Part model, mm, in its own coordinate system. A direction names the side the tool comes from. Coordinates: 2 decimals unless noted, no trailing zeros. Order: outer loops, then holes, each group sorted by start corner. A loop starts at its lowest first (then second) coordinate and runs counter-clockwise, first axis right, second up. Notation, with made-up numbers: (-33, 63) - (19, 63) arc R13 cw to (19, 82) - close; hole circle Ø4 at (84.25, -13.5). An arc over 180 degrees is marked (long way). Use a Markdown table: item, result. Add a question column.
1) Drop flat-ended pins along their axis: P1, Ø1, axis at y = 1.5, z = -1.5, coming from the -X side; P2, Ø3, axis at x = -2.5, y = -2, coming from the -Z side; P3, Ø5, axis at y = 3.5, z = -2, coming from the +X side. Give the stop position or say it passes through.
2) Wall check: L1, parallel to Z at x = 4.5, y = -4.5; L2, parallel to Z at x = -4, y = 2.5; L3, parallel to Z at x = -6.75, y = 1.25. Give the ranges that are in metal, low to high. Write a range as [from, to].
3) Two-plate mould, pull along Z, no slides. Class faces 5 (the face through (0, -5.5, -3)), 6 (the face through (4.52, -1.15, -6)), 7 (the face through (7.324, 0.077, -4.541)): +Z half, -Z half, draft (parallel to the pull), parting line (faces both ways), or undercut.
4) Tool access for faces 1 (the face through (-1.08, 4.88, -12.48)), 2 (the face through (-9.866, -2.835, -1.154)), 3 (the face through (9.884, -2.835, -1.154)), 4 (the face through (3.233, 1.341, -9.986)): list every direction of +Z, -Z, +X, -X, +Y, -Y with a clear straight run to the whole face (end or side of a thin tool).
5) Saw through at B-B on z = -4.75. List the corners of the cut face in (x, y), then the cut area to 3 significant figures.
6) Saw through at A-A on z = -1.5. List the corners of the cut face in (x, y).
```python
from build123d import *

# Parameters (mm, degrees)
Y_KSEKLIK_EKSTR_ZYON1_DEPTH = 5.5
IZIM4_R                     = 0.75
Y_KSEKLIK_EKSTR_ZYON2_DEPTH = 10.5
RADYUS1_R                   = 0.1
RADYUS2_R                   = 1.4


with BuildPart() as part:
    # Çizim1 → Yükseklik-Ekstrüzyon1 (new, symmetric)
    with BuildSketch(Plane(origin=(0, 0, 0), x_dir=(1, 0, 0), z_dir=(0, 1, 0))):
        Polygon((-9.25, 0), (9.25, 0), (9.25, 3), (5.5, 6), (-5.5, 6), (-9.25, 3), align=None)
    extrude(amount=Y_KSEKLIK_EKSTR_ZYON1_DEPTH, both=True)

    # Çizim2 → Döndür1 (revolve)
    with BuildSketch(Plane(origin=(0, 0, 0), x_dir=(1, 0, 0), z_dir=(0, 1, 0))):
        with BuildLine():
            Line((0, 6), (0, 13.8))
            Line((0, 13.8), (4.5, 13.8))
            Line((4.5, 13.8), (4.5, 14))
            Line((4.5, 14), (5, 14))
            Line((5, 14), (5, 11))
            Line((5, 11), (3.5, 11))
            Line((3.5, 11), (3.5, 9))
            ThreePointArc((3.5, 9), (3.465409062, 7.321803021), (4.5, 6))
            Line((4.5, 6), (0, 6))
        make_face()
    revolve(axis=Axis((0, 0, 0), (0, 0, -1)))

    # Çizim3 → Döndür2 (revolve)
    with BuildSketch(Plane(origin=(0, 0, 0), x_dir=(1, 0, 0), z_dir=(0, 1, 0))):
        with BuildLine():
            Line((0, 13.8), (4.75, 13.8))
            Line((4.75, 13.8), (4.75, 14))
            ThreePointArc((4.75, 14), (2.417928436, 14.654887588), (0, 14.8))
            Line((0, 14.8), (0, 13.8))
        make_face()
    revolve(axis=Axis((0, 0, 0), (0, 0, -1)))

    # Çizim4 → Yükseklik-Ekstrüzyon2 (add, symmetric)
    with BuildSketch(Plane(origin=(0, 0, 0), x_dir=(0, 0, -1), z_dir=(1, 0, 0))):
        with Locations(Location((1.5, -3.5, 0), (0, 0, 180))):
            Circle(IZIM4_R)
    extrude(amount=Y_KSEKLIK_EKSTR_ZYON2_DEPTH, both=True)

    # Radyus1
    radyus1_edges = [part.edges().sort_by_distance(p)[0] for p in [
        (-5, 0, -11),
        (-5, 0, -14),
        (-4.75, 0, -14),
    ]]
    fillet(radyus1_edges, radius=RADYUS1_R)

    # Radyus2
    radyus2_edges = [part.edges().sort_by_distance(p)[0] for p in [
        (-9.25, 0, -3),
        (-5.5, 0, -6),
        (5.5, 0, -6),
        (9.25, 0, -3),
    ]]
    fillet(radyus2_edges, radius=RADYUS2_R)


solid = part.part
```
Results are:
| question | item | result |
|---|---|---|
| 1 | P1 | x = -9.25 |
| 1 | P2 | z = -14.75 |
| 1 | P3 | x = 9.25 |
| 2 | L1 | [-6, 0] |
| 2 | L2 | [-14.01, -11], [-6, 0] |
| 2 | L3 | [-5, 0] |
| 3 | face 5 | draft |
| 3 | face 6 | undercut |
| 3 | face 7 | -Z half |
| 4 | face 1 | -Z |
| 4 | face 2 | -X |
| 4 | face 3 | +X |
| 4 | face 4 | none |
| 5 | outline | (-7.06, -5.5) - (7.06, -5.5) - (7.06, 5.5) - (-7.06, 5.5) - close |
| 5 | area | 155 mm2 |
| 6 | outline | (-10.5, -4.25) - (-9.25, -4.25) - (-9.25, -5.5) - (9.25, -5.5) - (9.25, -4.25) - (10.5, -4.25) - (10.5, -2.75) - (9.25, -2.75) - (9.25, 5.5) - (-9.25, 5.5) - (-9.25, -2.75) - (-10.5, -2.75) - close |
